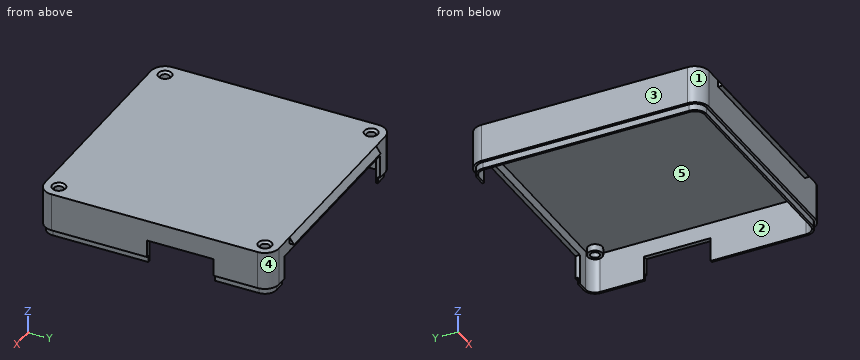
```python
from build123d import *

# Parameters (mm, degrees)
SKETCH1_R                = 3.25
BOSS_EXTRUDE1_DEPTH      = 3
BOSS_EXTRUDE1_2_DEPTH    = 3
BOSS_EXTRUDE1_3_DEPTH    = 3
BOSS_EXTRUDE1_4_DEPTH    = 3
BOSS_EXTRUDE2_DEPTH      = 2
BOSS_EXTRUDE3_DEPTH      = 20
SKETCH4_R                = 2
CUT_EXTRUDE1_DEPTH       = 5
CUT_EXTRUDE2_REACH       = 106.575
SKETCH6_W                = 82.790515713
SKETCH6_H                = 14.032058418
CUT_EXTRUDE3_REACH       = 106.575
SKETCH7_W                = 17
SKETCH7_H                = 29.705346692
CHAMFER1_SIZE            = 1
CUT_EXTRUDE4_DEPTH       = 3
BOSS_EXTRUDE4_DEPTH      = 65
BOSS_EXTRUDE4_DEPTH_BACK = 10


with BuildPart() as part:
    # Sketch1 → Boss-Extrude1 (new body)
    with BuildSketch(Plane(origin=(0, 0, 89.352648697), x_dir=(-1, 0, 0), z_dir=(0, 0, 1))):
        with Locations((-74.099367844, 104.955675546)):
            Circle(SKETCH1_R)
    extrude(amount=BOSS_EXTRUDE1_DEPTH)



with BuildPart() as body_2:
    # Sketch1 → Boss-Extrude1 2 (new body)
    with BuildSketch(Plane(origin=(0, 0, 89.352648697), x_dir=(-1, 0, 0), z_dir=(0, 0, 1))):
        with Locations((17.900817576, 104.955675546)):
            Circle(SKETCH1_R)
    extrude(amount=BOSS_EXTRUDE1_2_DEPTH)


with BuildPart() as body_3:
    # Sketch1 → Boss-Extrude1 3 (new body)
    with BuildSketch(Plane(origin=(0, 0, 89.352648697), x_dir=(-1, 0, 0), z_dir=(0, 0, 1))):
        with Locations((17.900817576, 12.955490126)):
            Circle(SKETCH1_R)
    extrude(amount=BOSS_EXTRUDE1_3_DEPTH)


with BuildPart() as body_4:
    # Sketch1 → Boss-Extrude1 4 (new body)
    with BuildSketch(Plane(origin=(0, 0, 89.352648697), x_dir=(-1, 0, 0), z_dir=(0, 0, 1))):
        with Locations((-74.099367844, 12.955490126)):
            Circle(SKETCH1_R)
    extrude(amount=BOSS_EXTRUDE1_4_DEPTH)


with BuildPart() as part_1:
    add(part.part)

    add(body_2.part)  # Boss-Extrude2 merges body 2

    add(body_3.part)  # Boss-Extrude2 merges body 3

    add(body_4.part)  # Boss-Extrude2 merges body 4
    # Sketch2 → Boss-Extrude2 (add)
    with BuildSketch(Plane(origin=(0, 0, 92.352648697), x_dir=(-1, 0, 0), z_dir=(0, 0, 1))):
        with BuildLine():
            Line((17.900817576, 109.242983141), (-74.099367844, 109.242983141))
            ThreePointArc((-74.099367844, 109.242983141), (-77.130952117, 107.987259819), (-78.386675439, 104.955675546))
            Line((-78.386675439, 104.955675546), (-78.386675439, 12.955490126))
            ThreePointArc((-78.386675439, 12.955490126), (-77.130952117, 9.923905853), (-74.099367844, 8.668182531))
            Line((-74.099367844, 8.668182531), (17.900817576, 8.668182531))
            ThreePointArc((17.900817576, 8.668182531), (20.93240185, 9.923905853), (22.188125171, 12.955490126))
            Line((22.188125171, 12.955490126), (22.188125171, 104.955675546))
            ThreePointArc((22.188125171, 104.955675546), (20.93240185, 107.987259819), (17.900817576, 109.242983141))
        make_face()
    extrude(amount=BOSS_EXTRUDE2_DEPTH)

    # Sketch3 → Boss-Extrude3 (add)
    with BuildSketch(Plane(origin=(0, 0, 94.352648697), x_dir=(-1, 0, 0), z_dir=(0, 0, 1))):
        with BuildLine():
            Line((17.900817576, 111.242983141), (-74.099367844, 111.242983141))
            ThreePointArc((-74.099367844, 111.242983141), (-78.54516568, 109.401473382), (-80.386675439, 104.955675546))
            Line((-80.386675439, 104.955675546), (-80.386675439, 12.955490126))
            ThreePointArc((-80.386675439, 12.955490126), (-78.54516568, 8.50969229), (-74.099367844, 6.668182531))
            Line((-74.099367844, 6.668182531), (17.900817576, 6.668182531))
            ThreePointArc((17.900817576, 6.668182531), (22.346615412, 8.50969229), (24.188125171, 12.955490126))
            Line((24.188125171, 12.955490126), (24.188125171, 104.955675546))
            ThreePointArc((24.188125171, 104.955675546), (22.346615412, 109.401473382), (17.900817576, 111.242983141))
        make_face()
        with BuildLine():
            Line((17.900817576, 109.242983141), (-74.099367844, 109.242983141))
            ThreePointArc((-74.099367844, 109.242983141), (-77.130952117, 107.987259819), (-78.386675439, 104.955675546))
            Line((-78.386675439, 104.955675546), (-78.386675439, 12.955490126))
            ThreePointArc((-78.386675439, 12.955490126), (-77.130952117, 9.923905853), (-74.099367844, 8.668182531))
            Line((-74.099367844, 8.668182531), (17.900817576, 8.668182531))
            ThreePointArc((17.900817576, 8.668182531), (20.93240185, 9.923905853), (22.188125171, 12.955490126))
            Line((22.188125171, 12.955490126), (22.188125171, 104.955675546))
            ThreePointArc((22.188125171, 104.955675546), (20.93240185, 107.987259819), (17.900817576, 109.242983141))
        make_face(mode=Mode.SUBTRACT)
    extrude(amount=-BOSS_EXTRUDE3_DEPTH)

    # Sketch4 → Cut-Extrude1 (cut)
    with BuildSketch(Plane(origin=(0, 0, 89.352648697), x_dir=(1, 0, 0), z_dir=(0, 0, -1))):
        with Locations((-17.900817576, 104.955675546)):
            Circle(SKETCH4_R)
        with Locations((74.099367844, 104.955675546)):
            Circle(SKETCH4_R)
        with Locations((74.099367844, 12.955490126)):
            Circle(SKETCH4_R)
        with Locations((-17.900817576, 12.955490126)):
            Circle(SKETCH4_R)
    extrude(amount=-CUT_EXTRUDE1_DEPTH, mode=Mode.SUBTRACT)

    # Sketch6 → Cut-Extrude2 (cut, up to next)
    with BuildSketch(Plane(origin=(0, -6.668182531, 0), x_dir=(1, 0, 0), z_dir=(0, 1, 0)), mode=Mode.PRIVATE) as cut_extrude2_sk1:
        with Locations((27.842461798, -80.850462516)):
            Rectangle(SKETCH6_W, SKETCH6_H)
    cut_extrude2_tool1 = extrude(cut_extrude2_sk1.sketch, amount=-CUT_EXTRUDE2_REACH, mode=Mode.PRIVATE) & part_1.part
    add(cut_extrude2_tool1.solids().sort_by_distance((27.842462, -6.668183, 80.850463))[0], mode=Mode.SUBTRACT)

    # Sketch7 → Cut-Extrude3 (cut, up to next)
    with BuildSketch(Plane(origin=(80.386675439, 0, 0), x_dir=(0, 0, -1), z_dir=(1, 0, 0)), mode=Mode.PRIVATE) as cut_extrude3_sk1:
        with Locations((-76.666440925, -47.447220968)):
            Rectangle(SKETCH7_W, SKETCH7_H)
    cut_extrude3_tool1 = extrude(cut_extrude3_sk1.sketch, amount=-CUT_EXTRUDE3_REACH, mode=Mode.PRIVATE) & part_1.part
    add(cut_extrude3_tool1.solids().sort_by_distance((80.386675, -47.447221, 76.666441))[0], mode=Mode.SUBTRACT)

    # Chamfer1
    chamfer1_edges = [part_1.edges().sort_by_distance(p)[0] for p in [
        (-19.900817576, -12.955490126, 94.352648697),
        (72.099367844, -12.955490126, 94.352648697),
        (72.099367844, -104.955675546, 94.352648697),
        (-19.900817576, -104.955675546, 94.352648697),
    ]]
    chamfer(chamfer1_edges, length=CHAMFER1_SIZE)

    # Sketch10 → Cut-Extrude4 (cut)
    with BuildSketch(Plane(origin=(0, 0, 74.352648697), x_dir=(-1, 0, 0), z_dir=(0, 0, -1))):
        with BuildLine():
            Line((-80.386675439, -12.955490126), (-80.386675439, -32.594547622))
            Line((-80.386675439, -32.594547622), (-80.386675439, -62.299894314))
            Line((-80.386675439, -62.299894314), (-80.386675439, -104.955675546))
            ThreePointArc((-80.386675439, -104.955675546), (-78.54516568, -109.401473382), (-74.099367844, -111.242983141))
            Line((-74.099367844, -111.242983141), (17.900817576, -111.242983141))
            ThreePointArc((17.900817576, -111.242983141), (22.346615412, -109.401473382), (24.188125171, -104.955675546))
            Line((24.188125171, -104.955675546), (24.188125171, -12.955490126))
            ThreePointArc((24.188125171, -12.955490126), (22.346615412, -8.50969229), (17.900817576, -6.668182531))
            Line((17.900817576, -6.668182531), (13.552796059, -6.668182531))
            Line((13.552796059, -6.668182531), (-69.237719654, -6.668182531))
            Line((-69.237719654, -6.668182531), (-74.099367844, -6.668182531))
            ThreePointArc((-74.099367844, -6.668182531), (-78.54516568, -8.50969229), (-80.386675439, -12.955490126))
        make_face()
        with BuildLine():
            Line((-79.286675439, -32.594547622), (-79.286675439, -62.299894314))
            Line((-79.286675439, -62.299894314), (-79.286675439, -104.955675546))
            ThreePointArc((-79.286675439, -104.955675546), (-77.76734822, -108.623655922), (-74.099367844, -110.142983141))
            Line((-74.099367844, -110.142983141), (17.900817576, -110.142983141))
            ThreePointArc((17.900817576, -110.142983141), (21.568797953, -108.623655922), (23.088125171, -104.955675546))
            Line((23.088125171, -104.955675546), (23.088125171, -12.955490126))
            ThreePointArc((23.088125171, -12.955490126), (21.568797953, -9.28750975), (17.900817576, -7.768182531))
            Line((17.900817576, -7.768182531), (13.552796059, -7.768182531))
            Line((13.552796059, -7.768182531), (-69.237719654, -7.768182531))
            Line((-69.237719654, -7.768182531), (-74.099367844, -7.768182531))
            ThreePointArc((-74.099367844, -7.768182531), (-77.76734822, -9.28750975), (-79.286675439, -12.955490126))
            Line((-79.286675439, -12.955490126), (-79.286675439, -32.594547622))
        make_face(mode=Mode.SUBTRACT)
    extrude(amount=-CUT_EXTRUDE4_DEPTH, mode=Mode.SUBTRACT)

    # Sketch11 → Boss-Extrude4 (add, two sides)
    with BuildSketch(Plane(origin=(0, 0, 0), x_dir=(0, 0, -1), z_dir=(1, 0, 0))) as boss_extrude4_sk:
        Polygon((-94.352648697, -6.668182531), (-91.352648697, -4.668182531), (-91.352648697, -6.668182531), align=None)
        Polygon((-94.352648697, -111.242983141), (-91.352648697, -111.242983141), (-91.352648697, -113.242983141), align=None)
    extrude(amount=BOSS_EXTRUDE4_DEPTH)
    extrude(boss_extrude4_sk.sketch, amount=-BOSS_EXTRUDE4_DEPTH_BACK)


solid = part_1.part
```
Input: part model. Units: mm. Frame: model coordinates. Face numbers are marked on the shaded views. A direction names the side the tool comes from. Round coordinates to 2 decimals unless told otherwise and drop trailing zeros. Order: outer loops, then holes, each group sorted by start corner. A loop starts at its lowest first (then second) coordinate and runs counter-clockwise, first axis right, second up. Notation, with made-up numbers: (-4, -39.75) - (33, -39.75) arc R14 ccw to (33, -16.75) - close; hole circle Ø6 at (29.25, 15). An arc over 180 degrees is marked (long way). Answer in a Markdown table with one row per item.
Item 1: Section query C-C (y = -65.5). Return the cut outline in (x, z), then the cut area to 3 significant figures.
Model answer:
| item | result |
|---|---|
| outline | (-24.19, 77.35) - (-23.09, 77.35) - (-23.09, 74.35) - (-22.19, 74.35) - (-22.19, 92.35) - (78.39, 92.35) - (78.39, 74.35) - (79.29, 74.35) - (79.29, 77.35) - (80.39, 77.35) - (80.39, 94.35) - (-24.19, 94.35) - close |
| area | 275 mm² |
Item 2: Reachability of the marked faces 4 and 5 from +Z, -Z, +X, -X, +Y, -Y: full face, straight path, thin tool, end or side. Return the list, or none.
Model answer:
| item | result |
|---|---|
| face 4 | +Z, -Z, +X, +Y |
| face 5 | -Z |
Item 3: Pin query (flat end, axial travel): pin 1 (2 mm diameter, centred on x = 18.5, y = -55.5, fed in from -Z); pin 2 (1 mm diameter, centred on x = 79.5, y = -44.5, fed in from -Z); pin 3 (2 mm diameter, centred on x = 79.5, z = 78.5, fed in from -Y); pin 4 (2.5 mm diameter, centred on x = -17.9, y = -104.96, fed in from -Z). Return the tip coordinate at first contact, or that it passes through.
Model answer:
| item | result |
|---|---|
| pin 1 | stops at z = 92.35 |
| pin 2 | stops at z = 85.17 |
| pin 3 | stops at y = -109.45 |
| pin 4 | passes through |
Item 4: Line query: line 1 (X direction, y = -48, z = 91.75); line 2 (Y direction, x = 8.5, z = 90.75); line 3 (Y direction, x = 44.5, z = 87). Output: solid intervals per line, ascending.
Model answer:
| item | result |
|---|---|
| line 1 | x = -24.19 to -22.19, 78.39 to 80.39 |
| line 2 | y = -111.24 to -109.24, -8.67 to -6.67 |
| line 3 | y = -111.24 to -109.24 |
Item 5: Section query A-A (z = 80). Return the cut outline in (x, y), then the cut area to 3 significant figures.
Model answer:
| item | result |
|---|---|
| outline | (-24.19, -104.96) arc R6.29 ccw to (-17.9, -111.24) - (74.1, -111.24) arc R6.29 ccw to (80.39, -104.96) - (80.39, -62.3) - (78.39, -62.3) - (78.39, -104.96) arc R4.29 cw to (74.1, -109.24) - (-17.9, -109.24) arc R4.29 cw to (-22.19, -104.96) - (-22.19, -12.96) arc R4.29 cw to (-17.9, -8.67) - (-13.55, -8.67) - (-13.55, -6.67) - (-17.9, -6.67) arc R6.29 ccw to (-24.19, -12.96) - close; (69.24, -8.67) - (74.1, -8.67) arc R4.29 cw to (78.39, -12.96) - (78.39, -32.59) - (80.39, -32.59) - (80.39, -12.96) arc R6.29 ccw to (74.1, -6.67) - (69.24, -6.67) - close |
| area | 577 mm² |
Item 6: Mould query, pull axis Y, two halves, no side actions, for the marked faces 1, 2 and 3. Classes: released by +Y, released by -Y, zero draft, split by the parting line, or undercut.
Model answer:
| item | result |
|---|---|
| face 1 | released by -Y |
| face 2 | undercut |
| face 3 | zero draft |
Item 7: Section query B-B (x = 30). Return the cut outline in (y, z).
Model answer:
| item | result |
|---|---|
| outline | (-113.24, 91.35) - (-111.24, 91.35) - (-111.24, 77.35) - (-110.14, 77.35) - (-110.14, 74.35) - (-109.24, 74.35) - (-109.24, 92.35) - (-8.67, 92.35) - (-8.67, 87.87) - (-6.67, 87.87) - (-6.67, 91.35) - (-4.67, 91.35) - (-6.67, 94.35) - (-111.24, 94.35) - close |
